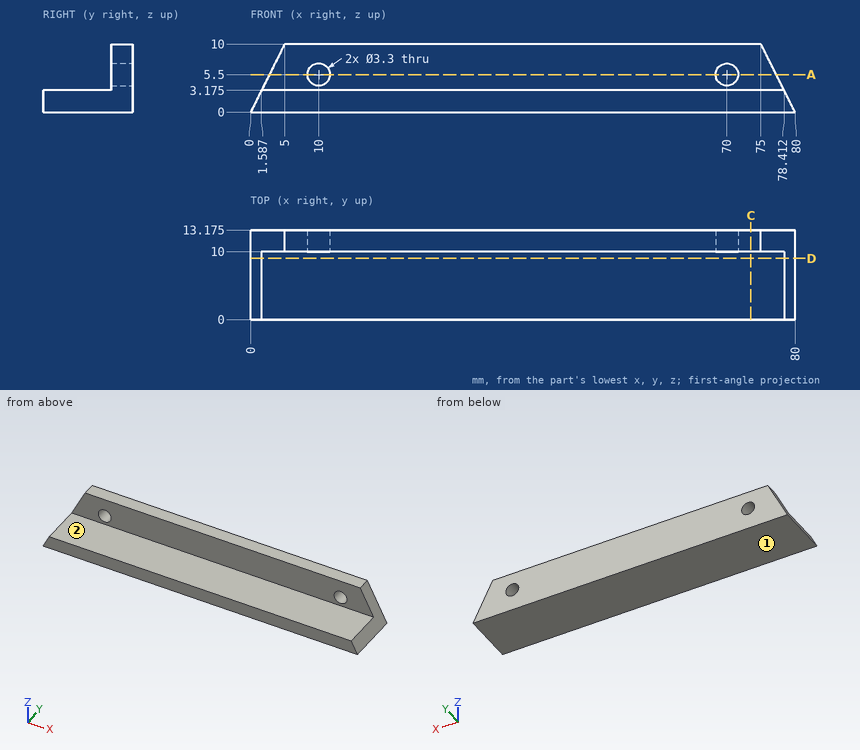
Could you check a few things on this drawing? It's one solid part, dimensions in mm from its lowest x, y, z. A direction names the side the tool comes from. Coordinates: 2 decimals unless noted, no trailing zeros. Order: outer loops, then holes, each group sorted by start corner. A loop starts at its lowest first (then second) coordinate and runs counter-clockwise, first axis right, second up. Notation, with made-up numbers: M -40,-2 L 1,-2 A36 cw 1,34 Z; hole C 71,88 d9. An arc over 180 degrees is marked long. Answer as a JSON object with one key per item and string values. Group by question number.
(1) Which directions (+Z, -Z, +X, -X, +Y, -Y) give clear straight access to the entire face, cutting with the end or side of a thin tool? Please do the marked faces 1 and 2.
(2) For pin 1 (4 mm diameter, centred on y = 11, z = 1, fed in from -X); pin 2 (2 mm diameter, centred on x = 69.5, z = 8, fed in from -Y); pin 3 (5 mm diameter, centred on y = 10.5, z = 6, fed in from +X), each with a flat end and sliding along its axis, tell me the tip position at first contact or that it passes through.
(3) Suppose I cut it at D-D, the plane y = 9. Please give me the cut outline in (x, z) (1 decimal).
(4) I need wall thicknesses on probe 1 along X at (y, z) = (10.95, 5.5); probe 2 along Z at (x, y) = (70, 12.2); probe 3 along Z at (x, y) = (38, 6) (1 decimal). Which ranges of each line are inside material? Lowest first, please.
(5) Suppose I cut it at C-C, the plane x = 73.5. Please give me the cut outline in (y, z) (1 decimal).
(6) Suppose I cut it at A-A, the plane z = 5.5. State how many separate pieces and enclosed holes the cut face has.
Values found:
{
 "1": {"face 1": "-Z, +X, -X, +Y, -Y", "face 2": "+Z, +X, -X, -Y"},
 "2": {"pin 1": "stops at x = 0", "pin 2": "stops at y = 10", "pin 3": "stops at x = 78.25"},
 "3": {"outline": "M 0,0 L 80,0 L 78.4,3.2 L 1.6,3.2 Z"},
 "4": {"probe 1": "x = 2.75 to 8.35, 11.65 to 68.35, 71.65 to 77.25", "probe 2": "z = 0 to 3.85, 7.15 to 10", "probe 3": "z = 0 to 3.2"},
 "5": {"outline": "M 0,0 L 13.2,0 L 13.2,10 L 10,10 L 10,3.2 L 0,3.2 Z"},
 "6": {"separate pieces": "3", "enclosed holes": "0"}
}
